Source: three-view drawing plus pictorial views. Frame: mm from the lowest corner of the part. A direction names the side the tool comes from. Round coordinates to 2 decimals unless told otherwise and drop trailing zeros. Order: outer loops, then holes, each group sorted by start corner. A loop starts at its lowest first (then second) coordinate and runs counter-clockwise, first axis right, second up. Notation, with made-up numbers: (68.5, 42.25) -> (99.5, 42.25) arc R28 ccw to (99.5, 63.25) -> close; hole circle Ø1 at (-22, -18.75). An arc over 180 degrees is marked (long way). Answer as CSV lines item,"result".
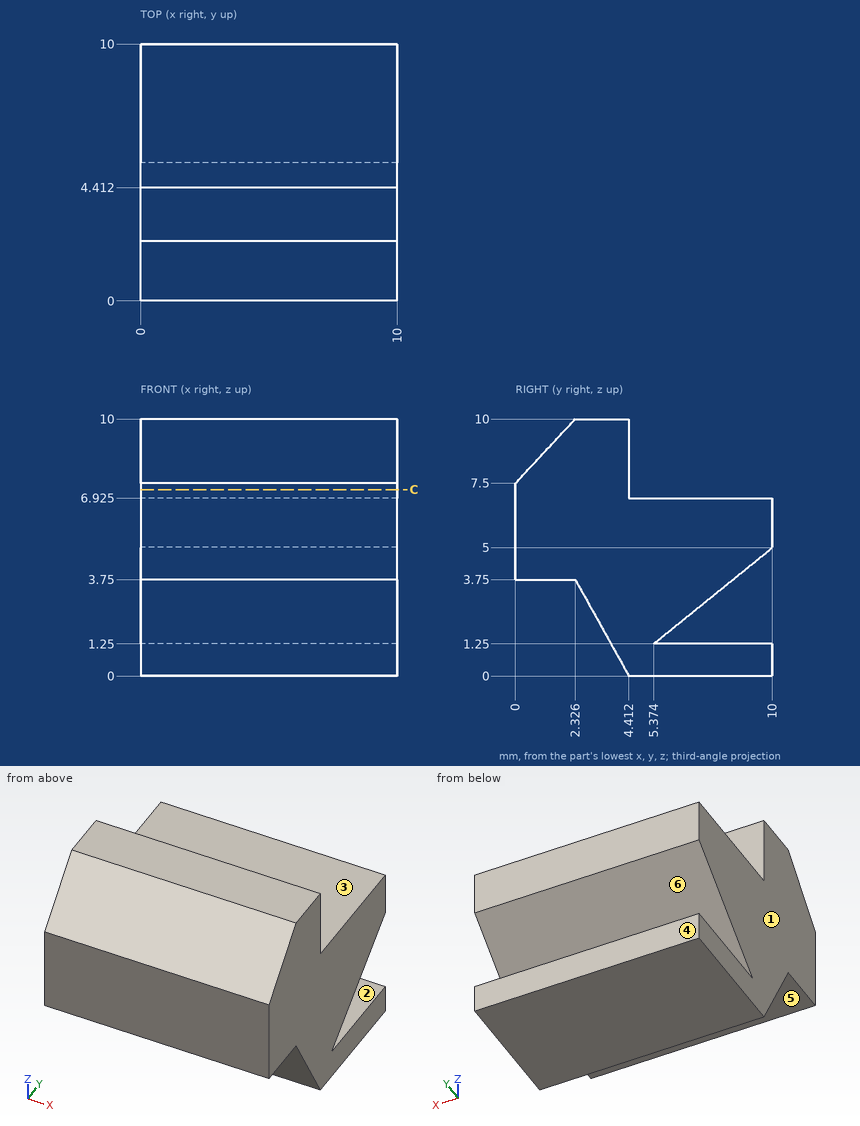
1. Section query C-C on z = 7.25. Return loops of the section in (x, y).
Results below:
outline,"(0, 0) -> (10, 0) -> (10, 4.41) -> (0, 4.41) -> close"
2. Line query: L1, parallel to Z at x = 5, y = 4.5 (1 decimal); L2, parallel to Y at x = 1.75, z = 7.25; L3, parallel to Y at x = 6.25, z = 3.25 (1 decimal). Output: solid intervals per line, ascending. Write a range as [from, to].
Results below:
L1,"[0, 6.9]"
L2,"[0, 4.41]"
L3,"[2.6, 7.8]"
3. Reachability of the marked faces 1, 2 and 3 from +Z, -Z, +X, -X, +Y, -Y: full face, straight path, thin tool, end or side. Return the list, or none.
Results below:
face 1,"+Z, -Z, -X, +Y, -Y"
face 2,"+X, -X, +Y"
face 3,"+Z, +X, -X, +Y"
4. Mould query, pull axis Z, two halves, no side actions, for the marked faces 4, 5 and 6. Classes: released by +Z, released by -Z, zero draft, split by the parting line, or undercut.
Results below:
face 4,"zero draft"
face 5,"released by -Z"
face 6,"undercut"
5. Pin query (flat end, axial travel): pin 1 (1 mm diameter, centred on y = 9, z = 5.5, fed in from -X); pin 2 (1.5 mm diameter, centred on x = 7.5, z = 3.5, fed in from +Y) (1 decimal); pin 3 (1.9 mm diameter, centred on x = 4, y = 0.5, fed in from -Z); pin 4 (3 mm diameter, centred on x = 6, y = 6.5, fed in from +Z) (1 decimal). Return the tip coordinate at first contact, or that it passes through.
Results below:
pin 1,"x = 0"
pin 2,"y = 9.1"
pin 3,"z = 3.75"
pin 4,"z = 6.9"
